Could you check a few things on this model? Use its own coordinates, in mm. Face numbers are marked on the shaded views. A direction names the side the tool comes from. Coordinates: 2 decimals unless noted, no trailing zeros. Loops run counter-clockwise (first coordinate to the right, second up) from the corner with the lowest first, then second, coordinate; pieces in that order, holes last. Notation, with made-up numbers: M 58,-19 L 74,-19 A32 cw 74,13 Z; hole C 34.25,-10 d8. An arc over 180 degrees is marked long. Use one line per item in the form item = value. Start each with the question number.
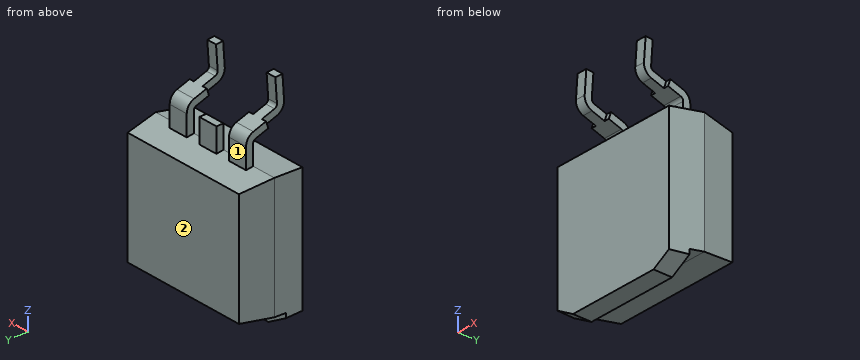
```python
from build123d import *

# Parameters (mm, degrees)
SKETCH1_W                  = 10.16
SKETCH1_H                  = 9.015
EXTRUDE1_DEPTH             = 2.385
EXTRUDE1_TAPER             = 7.5
EXTRUDE1_OTHER_WAY_DEPTH   = 2.385
EXTRUDE1_OTHER_WAY_TAPER   = 7.5
EXTRUDE2_REACH             = 9.198
EXTRUDE2_DIRECTION_2_REACH = 9.198
CUT_EXTRUDE5_REACH         = 11.097
EXTRUDE5_DEPTH             = 0.73
SKETCH29_W                 = 1.78
SKETCH29_H                 = 0.535
EXTRUDE6_DEPTH             = 0.73
CUT_EXTRUDE8_REACH         = 20.49
SKETCH34_W                 = 0.355
SKETCH34_H                 = 2.212694359


with BuildPart() as part:
    # Sketch1 → Extrude1 (new body)
    with BuildSketch(Plane(origin=(0, 0, 0), x_dir=(1, 0, 0), z_dir=(0, 1, 0))):
        Rectangle(SKETCH1_W, SKETCH1_H)
    extrude(amount=EXTRUDE1_DEPTH, taper=EXTRUDE1_TAPER)

    # Sketch1 → Extrude1 other way (add)
    with BuildSketch(Plane(origin=(0, 0, 0), x_dir=(1, 0, 0), z_dir=(0, 1, 0))):
        Rectangle(SKETCH1_W, SKETCH1_H)
    extrude(amount=-EXTRUDE1_OTHER_WAY_DEPTH, taper=EXTRUDE1_OTHER_WAY_TAPER)

    # Extrude2: up to this plane
    extrude2_end = Plane(origin=(5.08, 0, -4.5075), z_dir=(0.9914448613738104, -0.13052619222005188, 0))
    # Sketch2 → Extrude2 (add, up to the surface)
    with BuildSketch(Plane(origin=(0, 0, 0), x_dir=(0, 0, -1), z_dir=(1, 0, 0)), mode=Mode.PRIVATE) as extrude2_sk1:
        Polygon((4.5075, 0), (4.193508793, -2.385), (5.8475, -2.385), (5.8475, -0.99), (4.637835973, -0.99), align=None)
    extrude2_tool1 = split(extrude(extrude2_sk1.sketch, amount=EXTRUDE2_REACH, mode=Mode.PRIVATE), bisect_by=extrude2_end, keep=Keep.BOTH, mode=Mode.PRIVATE)
    add(extrude2_tool1.solids().sort_by_distance((0, -1.642965, -5.034325))[0])

    # Extrude2 direction 2: up to this plane
    extrude2_direction_2_end = Plane(origin=(-5.08, 0, -4.5075), z_dir=(-0.9914448613738104, -0.13052619222005188, 0))
    # Sketch2 → Extrude2 direction 2 (add, up to the surface)
    with BuildSketch(Plane(origin=(0, 0, 0), x_dir=(0, 0, -1), z_dir=(1, 0, 0)), mode=Mode.PRIVATE) as extrude2_direction_2_sk1:
        Polygon((4.5075, 0), (4.193508793, -2.385), (5.8475, -2.385), (5.8475, -0.99), (4.637835973, -0.99), align=None)
    extrude2_direction_2_tool1 = split(extrude(extrude2_direction_2_sk1.sketch, amount=-EXTRUDE2_DIRECTION_2_REACH, mode=Mode.PRIVATE), bisect_by=extrude2_direction_2_end, keep=Keep.BOTH, mode=Mode.PRIVATE)
    add(extrude2_direction_2_tool1.solids().sort_by_distance((0, -1.642965, -5.034325))[0])

    # Sketch27 → Cut-Extrude5 (cut, up to next)
    with BuildSketch(Plane(origin=(0, 2.385, 0), x_dir=(1, 0, 0), z_dir=(0, 1, 0)), mode=Mode.PRIVATE) as cut_extrude5_sk1:
        Polygon((3.449664027, 5.8475), (4.949664027, 5.8475), (4.949664027, 4.981474596), align=None)
    cut_extrude5_tool1 = extrude(cut_extrude5_sk1.sketch, amount=-CUT_EXTRUDE5_REACH, mode=Mode.PRIVATE) & part.part
    # Sketch27 → Cut-Extrude5 (cut, up to next)
    with BuildSketch(Plane(origin=(0, 2.385, 0), x_dir=(1, 0, 0), z_dir=(0, 1, 0)), mode=Mode.PRIVATE) as cut_extrude5_sk2:
        Polygon((-4.949664027, 4.981474596), (-3.449664027, 5.8475), (-4.949664027, 5.8475), align=None)
    cut_extrude5_tool2 = extrude(cut_extrude5_sk2.sketch, amount=-CUT_EXTRUDE5_REACH, mode=Mode.PRIVATE) & part.part
    add(cut_extrude5_tool1.solids().sort_by_distance((4.449664, 2.385, -5.558825))[0], mode=Mode.SUBTRACT)
    add(cut_extrude5_tool2.solids().sort_by_distance((-4.449664, 2.385, -5.558825))[0], mode=Mode.SUBTRACT)

    # Sketch28 → Extrude5 (add, symmetric)
    with BuildSketch(Plane(origin=(2.54, 0, 0), x_dir=(0, 0, -1), z_dir=(1, 0, 0))):
        with BuildLine():
            Line((-4.437065914, 0.535), (-5.972851804, 0.535))
            ThreePointArc((-5.972851804, 0.535), (-6.442417164, 0.383280011), (-6.734431244, -0.014511844))
            Line((-6.734431244, -0.014511844), (-7.366359813, -1.916829385))
            ThreePointArc((-7.366359813, -1.916829385), (-7.47136382, -2.054757056), (-7.638879483, -2.099348383))
            Line((-7.638879483, -2.099348383), (-9.378840143, -1.977678482))
            Line((-9.378840143, -1.977678482), (-9.416159857, -2.511375248))
            Line((-9.416159857, -2.511375248), (-7.676199197, -2.63304515))
            ThreePointArc((-7.676199197, -2.63304515), (-7.173652208, -2.499271168), (-6.858640187, -2.085488156))
            Line((-6.858640187, -2.085488156), (-6.226711617, -0.183170615))
            ThreePointArc((-6.226711617, -0.183170615), (-6.129373591, -0.05057333), (-5.972851804, 0))
            Line((-5.972851804, 0), (-4.437065914, 0))
            Line((-4.437065914, 0), (-4.437065914, 0.535))
        make_face()
    extrude5 = extrude(amount=EXTRUDE5_DEPTH, both=True)

    # Sketch29 → Extrude6 (add, symmetric)
    with BuildSketch(Plane(origin=(0, 0, 0), x_dir=(0, 0, -1), z_dir=(1, 0, 0))):
        with Locations((-5.327065914, 0.2675)):
            Rectangle(SKETCH29_W, SKETCH29_H)
    extrude(amount=EXTRUDE6_DEPTH, both=True)

    # Mirror1: Extrude5 across plane
    add(extrude5.mirror(Plane(origin=(0, 0, 0), x_dir=(0, 0, 1), z_dir=(1, 0, 0))))

    # Sketch34 → Cut-Extrude8 (cut, up to next)
    with BuildSketch(Plane(origin=(0, 3.589581516, 10.805847706), x_dir=(1, 0, 0), z_dir=(0, 0.3152500380612474, 0.9490086477489982)), mode=Mode.PRIVATE) as cut_extrude8_sk1:
        with Locations((3.0925, -4.245414402)):
            Rectangle(SKETCH34_W, SKETCH34_H)
    cut_extrude8_tool1 = extrude(cut_extrude8_sk1.sketch, amount=-CUT_EXTRUDE8_REACH, mode=Mode.PRIVATE) & part.part
    # Sketch34 → Cut-Extrude8 (cut, up to next)
    with BuildSketch(Plane(origin=(0, 3.589581516, 10.805847706), x_dir=(1, 0, 0), z_dir=(0, 0.3152500380612474, 0.9490086477489982)), mode=Mode.PRIVATE) as cut_extrude8_sk2:
        with Locations((1.9875, -4.245414402)):
            Rectangle(SKETCH34_W, SKETCH34_H)
    cut_extrude8_tool2 = extrude(cut_extrude8_sk2.sketch, amount=-CUT_EXTRUDE8_REACH, mode=Mode.PRIVATE) & part.part
    cut_extrude8_1 = cut_extrude8_tool1.solids().sort_by_distance((3.0925, -0.439353, 12.144215))[0]
    add(cut_extrude8_1, mode=Mode.SUBTRACT)
    cut_extrude8_2 = cut_extrude8_tool2.solids().sort_by_distance((1.9875, -0.439353, 12.144215))[0]
    add(cut_extrude8_2, mode=Mode.SUBTRACT)
    cut_extrude8 = cut_extrude8_1 + cut_extrude8_2  # Cut-Extrude8 as one shape, for the pattern or mirror that repeats it

    # Mirror2: Cut-Extrude8 across plane
    add(cut_extrude8.mirror(Plane(origin=(0, 0, 0), x_dir=(0, 0, 1), z_dir=(1, 0, 0))), mode=Mode.SUBTRACT)


solid = part.part
```
Item 1: I want a section at A-A (z = 5.75). Write out the boundary of the cut face in (x, y) (3 decimals).
Item 2: I'm going to push flat-ended pins straight in: P1, Ø0.7, axis at x = -0.5, z = 5, coming from the -Y side; P2, Ø1.5, axis at x = -0.5, z = 4.5, coming from the +Y side (3 decimals); P3, Ø1.6, axis at x = 2.5, z = 5.5, coming from the +Y side (3 decimals); P4, Ø1.3, axis at y = -1.5, z = 7.5, coming from the -X side (3 decimals). Where does each tip first touch, or does it pass through?
Item 3: Please list where these lines run through material, in increasing order: line 1 along X through (y, z) = (0.3, 5.5); line 2 along X through (y, z) = (-2.4, 8) (3 decimals); line 3 along Z through (x, y) = (3, -0.4).
Item 4: I want a section at B-B (z = 8.75). Write out the boundary of the cut face in (x, y) (3 decimals), plus the area to 3 significant figures.
Item 5: For the marked faces 1 and 2, which set-ups out of +Z, -Z, +X, -X, +Y, -Y let a thin tool reach every point of the face, with its end or its side?
Item 6: I want a section at C-C (y = -1.5). Count the separate pieces of the cut face and the enclosed holes in it, plus the area to 3 significant figures.
Worked answers:
q1.outline = M -3.27,0 L -1.81,0 L -1.81,0.535 L -3.27,0.535 Z; M -0.73,0 L 0.73,0 L 0.73,0.535 L -0.73,0.535 Z; M 1.81,0 L 3.27,0 L 3.27,0.535 L 1.81,0.535 Z
q2.P1 = 0
q2.P2 = 2.385
q2.P3 = 0.535
q2.P4 = -2.915
q3.line_1 = -3.27 to -1.81, -0.73 to 0.73, 1.81 to 3.27
q3.line_2 = -2.915 to -2.165, 2.165 to 2.915
q3.line_3 = -4.56 to 4.45, 6.3 to 6.86
q4.outline = M -2.915,-2.558 L -2.165,-2.558 L -2.165,-2.022 L -2.915,-2.022 Z; M 2.165,-2.558 L 2.915,-2.558 L 2.915,-2.022 L 2.165,-2.022 Z
q4.area = 0.804 mm²
q5.face_1 = +Z, +X, -X, +Y
q5.face_2 = +Z, -Z, +X, -X, +Y
q6.separate_pieces = 3
q6.enclosed_holes = 0
q6.area = 98.8 mm²
